```python
from build123d import *

# Parameters (mm, degrees)
EXTRUDE_1_DEPTH     = 15
SKETCH_2_R          = 1.5
CUT_EXTRUDE_1_DEPTH = 10
SKETCH_3_R          = 1.5
CUT_EXTRUDE_2_DEPTH = 10


with BuildPart() as part:
    # ｽｹｯﾁ1 → ﾎﾞｽ - 押し出し1 (new body)
    with BuildSketch(Plane.XY):
        Polygon((-4.461455774, 6.353305785), (-5.461455774, 6.353305785), (-5.461455774, -8.646694215), (9.538544226, -8.646694215), (9.538544226, -7.646694215), (-4.461455774, -7.646694215), align=None)
    extrude(amount=EXTRUDE_1_DEPTH)

    # ｽｹｯﾁ2 → ｶｯﾄ - 押し出し1 (cut)
    with BuildSketch(Plane.ZY.offset(5.461455774)):
        with Locations((7.5, -1.146694215)):
            Circle(SKETCH_2_R)
    extrude(amount=-CUT_EXTRUDE_1_DEPTH, mode=Mode.SUBTRACT)

    # ｽｹｯﾁ3 → ｶｯﾄ - 押し出し2 (cut)
    with BuildSketch(Plane.XZ.offset(8.646694215)):
        with Locations((2.038544226, 7.5)):
            Circle(SKETCH_3_R)
    extrude(amount=-CUT_EXTRUDE_2_DEPTH, mode=Mode.SUBTRACT)


solid = part.part
```
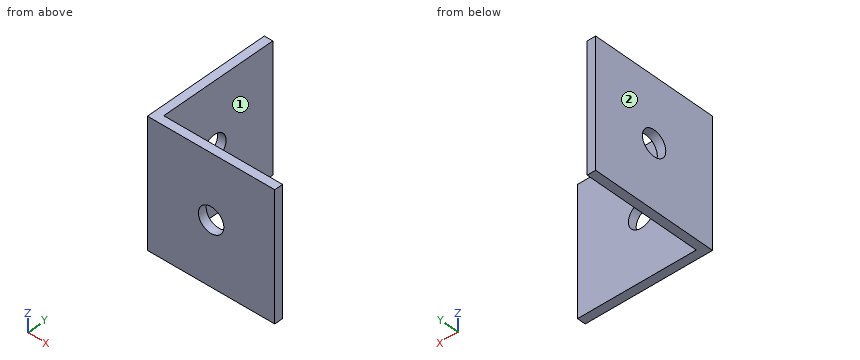
Can you work these out from the model? Positions are in its coordinate system, mm. Face numbers are marked on the shaded views. A direction names the side the tool comes from. Coordinates: 2 decimals unless noted, no trailing zeros. Write each loop counter-clockwise with the first axis right and the second up, starting at its lowest first coordinate (ties: lowest second). Pieces come first, ordered by that corner, then holes. Notation, with made-up numbers: M 35.5,74 L 80.5,74 A21 cw 80.5,92 Z; hole C 72.5,20.5 d6. An arc over 180 degrees is marked long. Write item = value, one per line. Start each with the question number.
Q1. On a 3-axis mill with a long thin cutter (end or side, diameter ignored), from which of +Z, -Z, +X, -X, +Y, -Y can I reach the whole of each face in a straight line? I mean the marked faces 1 and 2. Say none if no direction works.
Q2. I'm going to push flat-ended pins straight in: pin 1 (7 mm diameter, centred on x = 3.5, z = 9.5, fed in from +Y); pin 2 (7 mm diameter, centred on y = 0, z = 6, fed in from +X); pin 3 (1 mm diameter, centred on x = -3, y = -3.5, fed in from -Z). Where does each tip first touch, or does it pass through?
Q3. If we section it at A-A, the plane z = 7.5: Write out the boundary of the cut face in (x, y), then the cut area to 3 significant figures.
Q4. If we section it at C-C, the plane z = 12.5: Write out the boundary of the cut face in (x, y), then the cut area to 3 significant figures.
Q5. If I drill on L1, parallel to Y at x = 0.5, z = 6.5; L2, parallel to Y at x = -5, z = 7.5; L3, parallel to X at y = -6.75, z = 1, over which ranges is the centre line in solid material (lowest first)? Write a range as [from, to].
Q6. If we section it at B-B, the plane x = 2: Write out the boundary of the cut face in (y, z).
Q7. If we section it at D-D, the plane y = 2.25: Write out the boundary of the cut face in (x, z).
Check sheet entries:
q1.face_1 = +Z, -Z, +X, +Y
q1.face_2 = +Z, -Z, -X, +Y, -Y
q2.pin_1 = -7.65
q2.pin_2 = -4.46
q2.pin_3 = through
q3.outline = M -5.46,-8.65 L 0.54,-8.65 L 0.54,-7.65 L -4.46,-7.65 L -4.46,-2.65 L -5.46,-2.65 Z; M -5.46,0.35 L -4.46,0.35 L -4.46,6.35 L -5.46,6.35 Z; M 3.54,-8.65 L 9.54,-8.65 L 9.54,-7.65 L 3.54,-7.65 Z
q3.area = 23.0 mm²
q4.outline = M -5.46,-8.65 L 9.54,-8.65 L 9.54,-7.65 L -4.46,-7.65 L -4.46,6.35 L -5.46,6.35 Z
q4.area = 29.0 mm²
q5.L1 = [-8.65, -7.65]
q5.L2 = [-8.65, -2.65], [0.35, 6.35]
q5.L3 = [-5.46, -4.46]
q6.outline = M -8.65,0 L -7.65,0 L -7.65,6 L -8.65,6 Z; M -8.65,9 L -7.65,9 L -7.65,15 L -8.65,15 Z
q7.outline = M -5.46,0 L -4.46,0 L -4.46,15 L -5.46,15 Z
